from build123d import *

# Parameters (mm, degrees)
BOSS_EXTRUDE1_DEPTH                           = 76.2
CBORE_FOR_1_4_SOCKET_HEAD_CAP_SCREW1_AT_COUNT = 2
CBORE_FOR_1_4_SOCKET_HEAD_CAP_SCREW1_AT_PITCH = 50.8
F_7_16_0_4375_DIAMETER_HOLE1_D                = 11.1125


with BuildPart() as part:
    # Sketch2 → Boss-Extrude1 (new body)
    with BuildSketch(Plane(origin=(0, 0, 0), x_dir=(0, 0, -1), z_dir=(1, 0, 0))):
        Polygon((0, 0), (0, 44.45), (14.3002, 31.574042086), (14.3002, 12.875957914), align=None)
    extrude(amount=-BOSS_EXTRUDE1_DEPTH)

    # Sketch3 → CBORE for 1/4 Socket Head Cap Screw1 (revolve, cut)
    with BuildSketch(Plane(origin=(-63.5, 22.225, 0), x_dir=(0, -1, 0), z_dir=(1, 0, 0))):
        Polygon((0, 0), (0, 14.3002), (3.3782, 14.3002), (3.3782, 6.35), (5.55625, 6.35), (5.55625, 0.635), (6.19125, 0), align=None)
    cbore_for_1_4_socket_head_cap_screw1 = revolve(axis=Axis((-63.5, 22.225, 6.35), (0, 0, -1)), mode=Mode.SUBTRACT)

    # CBORE for 1/4 Socket Head Cap Screw1 at: CBORE for 1/4 Socket Head Cap Screw1 ×2
    with Locations(*[(i * CBORE_FOR_1_4_SOCKET_HEAD_CAP_SCREW1_AT_PITCH, 0, 0) for i in range(1, CBORE_FOR_1_4_SOCKET_HEAD_CAP_SCREW1_AT_COUNT)]):
        add(cbore_for_1_4_socket_head_cap_screw1, mode=Mode.SUBTRACT)

    # 7/16 (0.4375) Diameter Hole1 (through all)
    with Locations(Plane.XY):
        with Locations((-38.1, 22.225)):
            Hole(F_7_16_0_4375_DIAMETER_HOLE1_D / 2)


solid = part.part
Work out the finished part from the listing and answer in its coordinate system (mm). A direction names the side the tool comes from. Give positions to 0.01 mm unless a question says otherwise; leave off trailing zeros. Loops run counter-clockwise (first coordinate to the right, second up) from the corner with the lowest first, then second, coordinate; pieces in that order, holes last. Notation, with made-up numbers: (-1.5, -33) - (10.5, -33) arc R12 ccw to (10.5, -22) - close; hole circle Ø3 at (-31, 18.5). An arc over 180 degrees is marked (long way). Answer in a Markdown table with one row per item. Add a question column.
Q1. Each of these flat-tipped pins is pushed along its axis until it touches: P1, Ø6, axis at x = -40.5, z = -9.5, coming from the +Y side; P2, Ø4, axis at x = -35.5, z = -11.5, coming from the -Y side; P3, Ø5, axis at x = -15.5, y = 9.5, coming from the -Z side. Where does it stop, or does it pass through?
Q2. The part is cut by section C-C (x = -38.1). Determine the outline of the cut face in (y, z), and give its area (3 significant figures).
Q3. A tool of negligible diameter and unlimited length cuts with its end or side. For faces 1 (the flat face through (-37.57, 38.1, -7.05)), 2 (the flat face through (-10, 25, -6.35)), from which of +Z, -Z, +X, -X, +Y, -Y can it reach the whole face along a straight path? Write none if from no direction.
Q4. The part is cut by section D-D (y = 9). Determine the outline of the cut face in (x, z), and give its area (3 significant figures).
Q5. Consider line 1 along Y through (x, z) = (-63.5, -8.5); line 2 along Y through (x, z) = (-38.1, -3.5); line 3 along Z through (x, y) = (-65.5, 34.5). Determine where each line is inside the solid, lowest interval first.
Q6. The part is cut by section A-A (x = -63.5). Determine the outline of the cut face in (y, z) (3 decimals), and give its area (3 significant figures).
Q7. The part is cut by section B-B (z = -9.25). Determine the outline of the cut face in (x, y) (1 decimal), and give its area (3 significant figures).
Solution:
| question | item | result |
|---|---|---|
| 1 | P1 | stops at y = 38.6 |
| 1 | P2 | stops at y = 8.55 |
| 1 | P3 | stops at z = -13.33 |
| 2 | outline | (0, 0) - (12.88, -14.3) - (16.67, -14.3) - (16.67, 0) - close; (27.78, -14.3) - (31.57, -14.3) - (44.45, 0) - (27.78, 0) - close |
| 2 | area | 293 mm² |
| 3 | face 1 | -Z, +X, -X, +Y |
| 3 | face 2 | +Z |
| 4 | outline | (-76.2, -10) - (0, -10) - (0, 0) - (-76.2, 0) - close |
| 4 | area | 762 mm² |
| 5 | line 1 | y = 7.65 to 18.85, 25.6 to 36.8 |
| 5 | line 2 | y = 3.15 to 16.67, 27.78 to 41.3 |
| 5 | line 3 | z = -11.05 to 0 |
| 6 | outline | (0, 0) - (12.876, -14.3) - (18.847, -14.3) - (18.847, -6.35) - (16.669, -6.35) - (16.669, -0.635) - (16.034, 0) - close; (25.603, -14.3) - (31.574, -14.3) - (44.45, 0) - (28.416, 0) - (27.781, -0.635) - (27.781, -6.35) - (25.603, -6.35) - close |
| 6 | area | 327 mm² |
| 7 | outline | (-76.2, 8.3) - (0, 8.3) - (0, 36.1) - (-76.2, 36.1) - close; hole circle Ø6.8 at (-63.5, 22.2); hole circle Ø11.1 at (-38.1, 22.2); hole circle Ø6.8 at (-12.7, 22.2) |
| 7 | area | 1,950 mm² |
